Verification items for the finished model (mm, model axes). A direction names the side the tool comes from. Give positions to 0.01 mm unless a question says otherwise; leave off trailing zeros. Loops run counter-clockwise (first coordinate to the right, second up) from the corner with the lowest first, then second, coordinate; pieces in that order, holes last. Notation, with made-up numbers: M 30.5,-8.75 L 64.5,-8.75 A22 cw 64.5,15.25 Z; hole C 82.5,35.5 d9. An arc over 180 degrees is marked long. Answer in a Markdown table with one row per item.
```python
from build123d import *

# Parameters (mm, degrees)
F0_W      = 87.884
F0_H      = 162.56
F1_DEPTH  = 2.54
F2_W      = 3.81
F2_H      = 162.56
F3_DEPTH  = 19.05
F4_W      = 95.5031178892
F4_H      = 3.8138817525
F5_DEPTH  = 19.05
F8_D      = 1.27
F8_DEPTH  = 3.81
F8_TIP    = 0.3815464931
F9_D      = 1.27
F9_DEPTH  = 3.81
F9_TIP    = 0.3815464931
F11_D     = 1.27
F11_DEPTH = 3.81
F11_TIP   = 0.3815464931


with BuildPart() as f1:
    # F0 (on Top) → F1 (new body)
    with BuildSketch(Plane.XY):
        Rectangle(F0_W, F0_H)
    extrude(amount=F1_DEPTH)

    # F2 (on Top) → F3 (join)
    with BuildSketch(Plane.XY):
        with Locations((-45.847, 0)):
            Rectangle(F2_W, F2_H)
        with Locations((45.847, 0)):
            Rectangle(F2_W, F2_H)
    extrude(amount=F3_DEPTH)

    # F4 (on Top) → F5 (join)
    with BuildSketch(Plane.XY):
        with Locations((0.0004451722, -83.1869408762)):
            Rectangle(F4_W, F4_H)
    extrude(amount=F5_DEPTH)

    # F8
    with Locations(Plane.YZ.offset(47.752)):
        with Locations((-12.7, 16.51), (0, 16.51), (12.7, 16.51), (25.4, 16.51), (38.1, 16.51), (50.8, 16.51), (63.5, 16.51), (-25.4, 16.51), (-38.1, 16.51), (-50.8, 16.51), (-63.5, 16.51), (-76.2, 16.51)):
            Hole(F8_D / 2, depth=F8_DEPTH)
            with Locations((0, 0, -(F8_DEPTH + F8_TIP / 2))):  # 118° drill point
                Cone(0, F8_D / 2, F8_TIP, mode=Mode.SUBTRACT)

    # F9
    with Locations(Plane(origin=(-47.752, 0, 0), x_dir=(0, -1, 0), z_dir=(-1, 0, 0))):
        with Locations((-63.5, 16.51), (-50.8, 16.51), (-38.1, 16.51), (-12.7, 16.51), (0, 16.51), (-25.4, 16.51), (12.7, 16.51), (25.4, 16.51), (38.1, 16.51), (50.8, 16.51), (63.5, 16.51), (76.2, 16.51)):
            Hole(F9_D / 2, depth=F9_DEPTH)
            with Locations((0, 0, -(F9_DEPTH + F9_TIP / 2))):  # 118° drill point
                Cone(0, F9_D / 2, F9_TIP, mode=Mode.SUBTRACT)

    # F11
    with Locations(Plane.XZ.offset(85.0938817525)):
        with Locations((-38.1, 16.51), (-25.4, 16.51), (-12.7, 16.51), (0, 16.51), (12.7, 16.51), (25.4, 16.51), (38.1, 16.51)):
            Hole(F11_D / 2, depth=F11_DEPTH)
            with Locations((0, 0, -(F11_DEPTH + F11_TIP / 2))):  # 118° drill point
                Cone(0, F11_D / 2, F11_TIP, mode=Mode.SUBTRACT)


solid = f1.part
```
Item 1: Scan lines: L1, parallel to Z at x = 46.5, y = -38.1 (3 decimals); L2, parallel to X at y = 72, z = 5.5; L3, parallel to Y at x = -27, z = 4. Record each from-to range of solid material in increasing order. Write a range as [from, to].
Reported:
| item | result |
|---|---|
| L1 | z = [0, 15.875], [17.145, 19.05] |
| L2 | x = [-47.75, -43.94], [43.94, 47.75] |
| L3 | y = [-85.09, -81.28] |
Item 2: Sectioned sample at C-C (x = -4). Record the cut outline in (y, z), and give its area (3 significant figures).
Reported:
| item | result |
|---|---|
| outline | M -85.09,0 L 81.28,0 L 81.28,2.54 L -81.28,2.54 L -81.28,19.05 L -85.09,19.05 Z |
| area | 486 mm^2 |
Item 3: Release check for a two-part mould opening along X. For faces 3 (the flat face through (-1, -81.28, 11)), 4 (the flat face through (47.752, -83, 9)), 5 (the flat face through (-1, -1, 0)), 6 (the flat face through (-43.942, -1, 11)) record: released by +X, released by -X, zero draft, split by the parting line, or undercut.
Reported:
| item | result |
|---|---|
| face 3 | undercut |
| face 4 | released by +X |
| face 5 | zero draft |
| face 6 | undercut |
Item 4: Sectioned sample at B-B (y = 9). Record the cut outline in (x, z).
Reported:
| item | result |
|---|---|
| outline | M -47.75,0 L 47.75,0 L 47.75,19.05 L 43.94,19.05 L 43.94,2.54 L -43.94,2.54 L -43.94,19.05 L -47.75,19.05 Z |
Item 5: Go/stop test with flat-tipped pins: pin 1 (1.5 mm diameter, centred on x = -25.4, z = 16.51, fed in from +Y); pin 2 (1 mm diameter, centred on y = -38.1, z = 16.51, fed in from -X); pin 3 (10 mm diameter, centred on x = 27.5, y = 12.5, fed in from +Z). Record where each tip stops, or that it passes through.
Reported:
| item | result |
|---|---|
| pin 1 | stops at y = -81.28 |
| pin 2 | passes through |
| pin 3 | stops at z = 2.54 |
Item 6: Tool access check on faces 1 (the flat face through (-1, 1, 2.54)), 2 (the flat face through (-47.751, -83, 9)). Record the directions out of +Z, -Z, +X, -X, +Y, -Y that give a thin tool (end or side, any length) a straight path to the whole face; none if there is none.
Reported:
| item | result |
|---|---|
| face 1 | +Z, +Y |
| face 2 | +Z, -Z, -X, +Y, -Y |
